```python
from build123d import *

# Parameters (mm, degrees)
SALIENTE_EXTRUIR2_DEPTH     = 9
SALIENTE_EXTRUIR4_START     = -18
SALIENTE_EXTRUIR4_DEPTH     = 18
CORTAR_EXTRUIR3_DEPTH       = 81.972689334
CORTAR_EXTRUIR3_DEPTH_BACK  = 81.972689334
CROQUIS8_W                  = 8.024298647
CROQUIS8_H                  = 2.298422897
SALIENTE_EXTRUIR5_START     = -18
SALIENTE_EXTRUIR5_DEPTH     = 18
SALIENTE_EXTRUIR6_DEPTH     = 18
SALIENTE_EXTRUIR7_START     = -18
SALIENTE_EXTRUIR7_DEPTH     = 18
CORTAR_EXTRUIR5_DEPTH       = 118.18938142
CORTAR_EXTRUIR5_DEPTH_BACK  = 118.18938142
CROQUIS13_R                 = 1.5
CROQUIS14_R                 = 1.5
CORTAR_EXTRUIR7_DEPTH       = 4
CROQUIS15_R                 = 1.5
CORTAR_EXTRUIR8_DEPTH       = 97.711059211
CROQUIS16_R                 = 1.5
CORTAR_EXTRUIR9_DEPTH       = 97.711059211
CORTAR_EXTRUIR10_DEPTH      = 101.245514063
CORTAR_EXTRUIR10_DEPTH_BACK = 101.245514063
CROQUIS17_W                 = 15.073627069
CROQUIS17_H                 = 8.059357869


with BuildPart() as part:
    # Croquis1 → Saliente-Extruir2 (new, symmetric)
    with BuildSketch(Plane.XY):
        with BuildLine():
            ThreePointArc((-66.012618404, 0.60672559), (4.861867519, -30.780766865), (41.832299444, 37.348188804))
            ThreePointArc((41.832299444, 37.348188804), (33.631578066, 42.234206494), (28.745560376, 34.033485116))
            ThreePointArc((28.745560376, 34.033485116), (0.508301336, -18.002016476), (-53.624180056, 5.97110769))
            ThreePointArc((-53.624180056, 5.97110769), (-62.50059028, 9.483135814), (-66.012618404, 0.60672559))
        make_face()
        with BuildLine():
            ThreePointArc((37.954747128, 36.366054378), (34.613712492, 38.356654178), (32.623112692, 35.015619542))
            ThreePointArc((32.623112692, 35.015619542), (1.798246872, -21.788312888), (-57.294828456, 4.381661142))
            ThreePointArc((-57.294828456, 4.381661142), (-60.911143732, 5.812487414), (-62.341970004, 2.196172138))
            ThreePointArc((-62.341970004, 2.196172138), (3.571921983, -26.994470453), (37.954747128, 36.366054378))
        make_face(mode=Mode.SUBTRACT)
    extrude(amount=SALIENTE_EXTRUIR2_DEPTH, both=True)

    # Croquis7 → Saliente-Extruir4 (add)
    with BuildSketch(Plane(origin=(0, 0, -9), x_dir=(-1, 0, 0), z_dir=(0, 0, -1)).offset(SALIENTE_EXTRUIR4_START)):
        with BuildLine():
            Line((54.145016493, 6.946132565), (38.567143253, 6.946132565))
            Line((38.567143253, 6.946132565), (38.567143253, 3.946132565))
            Line((38.567143253, 3.946132565), (43.567143253, 3.946132565))
            ThreePointArc((43.567143253, 3.946132565), (48.081738335, 1.095186137), (47.447985926, -4.206494934))
            ThreePointArc((47.447985926, -4.206494934), (50.884688207, 0.670758181), (53.624180056, 5.97110769))
            ThreePointArc((53.624180056, 5.97110769), (53.864605301, 6.469299926), (54.145016493, 6.946132565))
        make_face()
    extrude(amount=SALIENTE_EXTRUIR4_DEPTH)

    # Croquis8 → Cortar-Extruir3 (cut, two sides: drawn at the far end of the back side and taken through both)
    with BuildSketch(Plane(origin=(0, 0, -9), x_dir=(-1, 0, 0), z_dir=(0, 0, -1)).offset(-CORTAR_EXTRUIR3_DEPTH_BACK)):
        with Locations((58.157165816, 8.095344014)):
            Rectangle(CROQUIS8_W, CROQUIS8_H)
    extrude(amount=CORTAR_EXTRUIR3_DEPTH + CORTAR_EXTRUIR3_DEPTH_BACK, mode=Mode.SUBTRACT)

    # Croquis9 → Saliente-Extruir5 (add)
    with BuildSketch(Plane(origin=(0, 0, -9), x_dir=(-1, 0, 0), z_dir=(0, 0, -1)).offset(SALIENTE_EXTRUIR5_START)):
        with BuildLine():
            Line((78.728806569, 3.946132565), (78.728806569, 6.946132565))
            Line((78.728806569, 6.946132565), (65.491781967, 6.946132565))
            ThreePointArc((65.491781967, 6.946132565), (66.526259445, 4.041984592), (66.161494713, 0.980748601))
            ThreePointArc((66.161494713, 0.980748601), (68.00603961, 3.139763461), (70.728806569, 3.946132565))
            Line((70.728806569, 3.946132565), (78.728806569, 3.946132565))
        make_face()
    extrude(amount=SALIENTE_EXTRUIR5_DEPTH)

    # Croquis10 → Saliente-Extruir6 (add)
    with BuildSketch(Plane.XY.offset(9)):
        with BuildLine():
            Line((18.89630467, 56.388029989), (18.89630467, 21.388029989))
            Line((18.89630467, 21.388029989), (21.89630467, 21.388029989))
            Line((21.89630467, 21.388029989), (21.89630467, 29.388029989))
            ThreePointArc((21.89630467, 29.388029989), (24.089730114, 33.5260415), (28.745560376, 34.033485116))
            ThreePointArc((28.745560376, 34.033485116), (30.517183559, 40.465031841), (36.949638278, 42.233355414))
            Line((36.949638278, 42.233355414), (24.158212062, 45.48024401))
            ThreePointArc((24.158212062, 45.48024401), (22.528364866, 46.546057924), (21.89630467, 48.388029989))
            Line((21.89630467, 48.388029989), (21.89630467, 56.388029989))
            Line((21.89630467, 56.388029989), (18.89630467, 56.388029989))
        make_face()
    extrude(amount=-SALIENTE_EXTRUIR6_DEPTH)

    # Croquis12 → Saliente-Extruir7 (add)
    with BuildSketch(Plane(origin=(0, 0, -9), x_dir=(-1, 0, 0), z_dir=(0, 0, -1)).offset(SALIENTE_EXTRUIR7_START)):
        with BuildLine():
            Line((-41.832299444, 37.348188804), (-40.312576156, 43.348188804))
            ThreePointArc((-40.312576156, 43.348188804), (-39.483140086, 44.774662002), (-38.02482177, 45.546735616))
            Line((-38.02482177, 45.546735616), (-24.275894818, 48.452882358))
            ThreePointArc((-24.275894818, 48.452882358), (-22.565936721, 49.49874832), (-21.89630467, 51.388029989))
            Line((-21.89630467, 51.388029989), (-21.89630467, 59.388029989))
            Line((-21.89630467, 59.388029989), (-18.89630467, 59.388029989))
            Line((-18.89630467, 59.388029989), (-18.89630467, 21.388029989))
            Line((-18.89630467, 21.388029989), (-21.89630467, 21.388029989))
            Line((-21.89630467, 21.388029989), (-21.89630467, 29.388029989))
            ThreePointArc((-21.89630467, 29.388029989), (-24.089730114, 33.5260415), (-28.745560376, 34.033485116))
            Line((-28.745560376, 34.033485116), (-32.623112692, 35.015619542))
            ThreePointArc((-32.623112692, 35.015619542), (-34.613712492, 38.356654178), (-37.954747128, 36.366054378))
            Line((-37.954747128, 36.366054378), (-41.832299444, 37.348188804))
        make_face()
    extrude(amount=SALIENTE_EXTRUIR7_DEPTH)

    # Croquis13 → Cortar-Extruir5 (cut, two sides: drawn at the far end of the back side and taken through both)
    with BuildSketch(Plane(origin=(21.89630467, 0, 0), x_dir=(0, 0, -1), z_dir=(1, 0, 0)).offset(-CORTAR_EXTRUIR5_DEPTH_BACK)):
        with Locations(Location((0, 55.388029989, 0), (0, 0, 90))):
            Circle(CROQUIS13_R)
    extrude(amount=CORTAR_EXTRUIR5_DEPTH + CORTAR_EXTRUIR5_DEPTH_BACK, mode=Mode.SUBTRACT)

    # Croquis14 → Cortar-Extruir7 (cut, symmetric)
    with BuildSketch(Plane(origin=(21.89630467, 0, 0), x_dir=(0, 0, -1), z_dir=(1, 0, 0))):
        with Locations((0, 25.388029989)):
            Circle(CROQUIS14_R)
    extrude(amount=CORTAR_EXTRUIR7_DEPTH, both=True, mode=Mode.SUBTRACT)

    # Croquis15 → Cortar-Extruir8 (cut, through all)
    with BuildSketch(Plane.XZ.offset(-3.946132565)):
        with Locations((-74.728806569, 0)):
            Circle(CROQUIS15_R)
    extrude(amount=-CORTAR_EXTRUIR8_DEPTH, mode=Mode.SUBTRACT)

    # Croquis16 → Cortar-Extruir9 (cut, through all)
    with BuildSketch(Plane.XZ.offset(-3.946132565)):
        with Locations(Location((-41.067143253, 0, 0), (0, 0, 270))):
            Circle(CROQUIS16_R)
    extrude(amount=-CORTAR_EXTRUIR9_DEPTH, mode=Mode.SUBTRACT)

    # Croquis17 → Cortar-Extruir10 (cut, two sides: drawn at the far end of the back side and taken through both)
    with BuildSketch(Plane.XY.offset(9).offset(-CORTAR_EXTRUIR10_DEPTH_BACK)):
        with Locations((-57.954968433, 10.9758115)):
            Rectangle(CROQUIS17_W, CROQUIS17_H)
    extrude(amount=CORTAR_EXTRUIR10_DEPTH + CORTAR_EXTRUIR10_DEPTH_BACK, mode=Mode.SUBTRACT)


solid = part.part
```
Check sheet for the modelled part. Datum: model origin and axes. Units: mm. A direction names the side the tool comes from. Give positions to 0.01 mm unless a question says otherwise; leave off trailing zeros. Loops run counter-clockwise (first coordinate to the right, second up) from the corner with the lowest first, then second, coordinate; pieces in that order, holes last. Notation, with made-up numbers: M 39.25,67 L 78.25,67 A25 cw 78.25,105 Z; hole C 50,-1.5 d8. An arc over 180 degrees is marked long. Answer in a Markdown table with one row per item.
1) Tool access check on faces 3 (the face through (20, 21.388, 0)), 4 (the face through (20.417, 23.924, 0.325)), 5 (the face through (18.896, 41, 0)), 6 (the face through (24.034, 33.487, 0.126)). Record the directions out of +Z, -Z, +X, -X, +Y, -Y that give a thin tool (end or side, any length) a straight path to the whole face; none if there is none.
Solutions:
| item | result |
|---|---|
| face 3 | +Z, -Z, -X |
| face 4 | -X |
| face 5 | +Z, -Z, -X, +Y |
| face 6 | +Z, -Z |
2) Mould release check, pull along Z, two halves, no side actions. Record for faces 1 (the face through (-73.298, 5.425, 0.451)), 2 (the face through (21.896, 23.6, 0.1)): released by +Z, released by -Z, zero draft, split by the parting line, or undercut.
Solutions:
| item | result |
|---|---|
| face 1 | undercut |
| face 2 | zero draft |
3) Cross-section at D-D (y = 32). Enter the section's corners in (x, z).
Solutions:
| item | result |
|---|---|
| outline | M 18.9,-9 L 22.63,-9 L 22.63,9 L 18.9,9 Z; M 29.21,-9 L 33.28,-9 L 33.28,9 L 29.21,9 Z; M 38.87,-9 L 42.92,-9 L 42.92,9 L 38.87,9 Z |
4) Cross-section at A-A (y = -1.5). Enter the section's corners in (x, z), plus the area to 3 significant figures.
Solutions:
| item | result |
|---|---|
| outline | M -65.05,-9 L -60.57,-9 L -60.57,9 L -65.05,9 Z; M -54.25,-9 L -48.55,-9 L -48.55,9 L -54.25,9 Z; M 22.34,-9 L 27.11,-9 L 27.11,9 L 22.34,9 Z; M 33.43,-9 L 37.91,-9 L 37.91,9 L 33.43,9 Z |
| area | 350 mm^2 |
5) Depth check by flat-ended pin: pin 1 (6 mm diameter, centred on x = -21, z = 1.5, fed in from -Y); pin 2 (1.5 mm diameter, centred on x = 20.5, z = 0, fed in from -Y); pin 3 (4 mm diameter, centred on x = -9.5, z = -4, fed in from -Y); pin 4 (1.5 mm diameter, centred on x = -57.5, y = -4.5, fed in from -Z). Enter the tip coordinate at first touch or a pass-through.
Solutions:
| item | result |
|---|---|
| pin 1 | stops at y = -33.66 |
| pin 2 | stops at y = -23.12 |
| pin 3 | stops at y = -33.8 |
| pin 4 | passes through |
6) Cross-section at B-B (x = -22.5). Enter the section's corners in (y, z).
Solutions:
| item | result |
|---|---|
| outline | M -33.13,-9 L -29.08,-9 L -29.08,9 L -33.13,9 Z; M -23.49,-9 L -19.41,-9 L -19.41,9 L -23.49,9 Z |
7) Thickness scan on line 1 (X direction, y = 2, z = -1.75); line 2 (Y direction, x = 23.5, z = 2); line 3 (Y direction, x = 20.5, z = 3). Record the ranges inside material, lowest first.
Solutions:
| item | result |
|---|---|
| line 1 | x = -66.77 to -62.26, -56.18 to -47.53, 24.52 to 29.05, 35.12 to 39.46 |
| line 2 | y = -20.18 to -14.77, -6.63 to 0.27, 33.06 to 48.73 |
| line 3 | y = -22.57 to -17.48, -10 to -3.97, 21.39 to 59.39 |
8) Cross-section at C-C (z = 3.25). Enter the section's corners in (x, y), plus the area to 3 significant figures.
Solutions:
| item | result |
|---|---|
| outline | M -78.73,3.95 L -70.73,3.95 A5 cw -66.16,0.98 A6.75 ccw -66.01,0.61 A57.15 ccw 41.83,37.35 L 40.31,43.35 A3 ccw 38.02,45.55 L 24.28,48.45 A3 cw 21.9,51.39 L 21.9,59.39 L 18.9,59.39 L 18.9,21.39 L 21.9,21.39 L 21.9,29.39 A5 cw 28.75,34.03 A43.65 cw -47.45,-4.21 A5 cw -43.57,3.95 L -38.57,3.95 L -38.57,6.95 L -78.73,6.95 Z; hole M -62.34,2.2 A53.15 ccw 37.95,36.37 A2.75 ccw 32.62,35.02 A47.65 cw -57.29,4.38 A2.75 ccw Z |
| area | 1,670 mm^2 |
